Work out the finished part from the listing and answer in its coordinate system (mm). A direction names the side the tool comes from. Give positions to 0.01 mm unless a question says otherwise; leave off trailing zeros. Loops run counter-clockwise (first coordinate to the right, second up) from the corner with the lowest first, then second, coordinate; pieces in that order, holes last. Notation, with made-up numbers: M 31.5,50.25 L 68.5,50.25 A24 ccw 68.5,78.25 Z; hole C 71.5,-26 d6. An arc over 180 degrees is marked long. Use a Markdown table: item, result.
```python
from build123d import *

# Parameters (mm, degrees)
SKETCH1_W           = 104.902
SKETCH1_H           = 114.3
BOSS_EXTRUDE1_DEPTH = 10.16
SKETCH2_W           = 35.56
SKETCH2_H           = 45.72
CUT_EXTRUDE1_DEPTH  = 8.255
SKETCH3_W           = 53.848
SKETCH3_H           = 101.6
CUT_EXTRUDE2_DEPTH  = 8.255
CUT_EXTRUDE3_DEPTH  = 8.255
FILLET1_R           = 5.08
CHAMFER1_SIZE       = 2.54


with BuildPart() as part:
    # Sketch1 → Boss-Extrude1 (new body)
    with BuildSketch(Plane(origin=(0, 0, 0), x_dir=(1, 0, 0), z_dir=(0, 1, 0))):
        Rectangle(SKETCH1_W, SKETCH1_H)
    extrude(amount=BOSS_EXTRUDE1_DEPTH)

    # Sketch2 → Cut-Extrude1 (cut)
    with BuildSketch(Plane(origin=(0, 10.16, 0), x_dir=(1, 0, 0), z_dir=(0, 1, 0))):
        with Locations((-29.591, 29.21)):
            Rectangle(SKETCH2_W, SKETCH2_H)
    extrude(amount=-CUT_EXTRUDE1_DEPTH, mode=Mode.SUBTRACT)

    # Sketch3 → Cut-Extrude2 (cut)
    with BuildSketch(Plane(origin=(0, 10.16, 0), x_dir=(1, 0, 0), z_dir=(0, 1, 0))):
        with Locations((20.447, 1.27)):
            Rectangle(SKETCH3_W, SKETCH3_H)
    extrude(amount=-CUT_EXTRUDE2_DEPTH, mode=Mode.SUBTRACT)

    # Sketch4 → Cut-Extrude3 (cut)
    with BuildSketch(Plane(origin=(0, 10.16, 0), x_dir=(1, 0, 0), z_dir=(0, 1, 0))):
        Polygon((1.143, -49.53), (13.843, -49.53), (33.528, -49.53), (43.688, -49.53), (43.688, -57.15), (33.528, -57.15), (15.4686, -57.15), (1.143, -57.15), align=None)
    extrude(amount=-CUT_EXTRUDE3_DEPTH, mode=Mode.SUBTRACT)

    # Fillet1
    fillet1_edges = [part.edges().sort_by_distance(p)[0] for p in [
        (-52.451, 5.08, -57.15),
        (52.451, 5.08, -57.15),
        (52.451, 5.08, 57.15),
        (-52.451, 5.08, 57.15),
    ]]
    fillet(fillet1_edges, radius=FILLET1_R)

    # Chamfer1
    chamfer1_edges = [part.edges().sort_by_distance(p)[0] for p in [
        (45.5295, 10.16, 57.15),
        (52.451, 10.16, 0),
        (-23.114, 10.16, 57.15),
        (0, 10.16, -57.15),
        (-52.451, 10.16, 0),
        (50.963102448, 10.16, -55.662102448),
        (-50.963102448, 10.16, -55.662102448),
        (-50.963102448, 10.16, 55.662102448),
        (50.963102448, 10.16, 55.662102448),
    ]]
    chamfer(chamfer1_edges, length=CHAMFER1_SIZE)


solid = part.part
```
(1) Given P1, Ø1.5, axis at x = 16.5, z = -6, coming from the +Y side (3 decimals); P2, Ø3, axis at x = 35.5, z = -22.5, coming from the -Y side; P3, Ø4, axis at x = 33, y = 7.5, coming from the +Z side; P4, Ø2.5, axis at y = 7, z = 54, coming from the +X side, each flat-ended and moving along its own axis, determine where each tip first touches the part or whether it passes through.
Entries:
| item | result |
|---|---|
| P1 | stops at y = 1.905 |
| P2 | stops at y = 0 |
| P3 | stops at z = -52.07 |
| P4 | stops at x = 52.41 |
(2) Consider probe 1 along X at (y, z) = (2.25, -34); probe 2 along Z at (x, y) = (-17, 5); probe 3 along X at (y, z) = (2.5, -4). Determine where each line is inside the solid, lowest interval first. Write a range as [from, to].
Entries:
| item | result |
|---|---|
| probe 1 | x = [-52.45, -47.37], [-11.81, -6.48], [47.37, 52.45] |
| probe 2 | z = [-57.15, -52.07], [-6.35, 57.15] |
| probe 3 | x = [-52.45, -6.48], [47.37, 52.45] |
(3) A cutting plane is placed at B-B (z = -29.5). Write down the section's boundary in (x, y) (3 decimals), and give its area (3 significant figures).
Entries:
| item | result |
|---|---|
| outline | M -52.451,0 L 52.451,0 L 52.451,7.62 L 49.911,10.16 L 47.371,10.16 L 47.371,1.905 L -6.477,1.905 L -6.477,10.16 L -11.811,10.16 L -11.811,1.905 L -47.371,1.905 L -47.371,10.16 L -49.911,10.16 L -52.451,7.62 Z |
| area | 321 mm² |
(4) A cutting plane is placed at D-D (x = 39). Write down the section's boundary in (y, z) (3 decimals).
Entries:
| item | result |
|---|---|
| outline | M 0,-57.15 L 7.62,-57.15 L 10.16,-54.61 L 10.16,-52.07 L 1.905,-52.07 L 1.905,57.15 L 0,57.15 Z |
(5) Which of the six approach directions +Z, -Z, +X, -X, +Y, -Y give full straight-line access (tool end or side, diameter ignored) to faces 1 (the flat face through (-51.2, 8.87, -0.73)), 2 (the flat face through (43.688, 6, 53)), 3 (the flat face through (-47.371, 6, -29))?
Entries:
| item | result |
|---|---|
| face 1 | +Z, -Z, -X, +Y |
| face 2 | +Z, +Y |
| face 3 | +Y |
(6) The mould has two halves that part along X. Classify faces 4 (the flat face through (-30, 6, -52.07)), 5 (the flat face through (45.5, 8.87, 55.9)), 6 (the flat face through (52.451, 4, 1)): released by +X, released by -X, zero draft, split by the parting line, or undercut.
Entries:
| item | result |
|---|---|
| face 4 | undercut |
| face 5 | zero draft |
| face 6 | released by +X |
(7) A cutting plane is placed at C-C (y = 4). Write down the section's boundary in (x, z), and give its area (3 significant figures).
Entries:
| item | result |
|---|---|
| outline | M -52.45,-52.07 A5.08 ccw -47.37,-57.15 L 47.37,-57.15 A5.08 ccw 52.45,-52.07 L 52.45,52.07 A5.08 ccw 47.37,57.15 L 43.69,57.15 L 43.69,49.53 L 47.37,49.53 L 47.37,-52.07 L -6.48,-52.07 L -6.48,49.53 L 1.14,49.53 L 1.14,57.15 L -47.37,57.15 A5.08 ccw -52.45,52.07 Z; hole M -47.37,-52.07 L -11.81,-52.07 L -11.81,-6.35 L -47.37,-6.35 Z |
| area | 4,550 mm² |
(8) A cutting plane is placed at A-A (x = -40). Write down the section's boundary in (y, z) (3 decimals).
Entries:
| item | result |
|---|---|
| outline | M 0,-57.15 L 7.62,-57.15 L 10.16,-54.61 L 10.16,-52.07 L 1.905,-52.07 L 1.905,-6.35 L 10.16,-6.35 L 10.16,54.61 L 7.62,57.15 L 0,57.15 Z |
